Input: part model. Units: mm. Frame: model coordinates. A direction names the side the tool comes from. Round coordinates to 2 decimals unless told otherwise and drop trailing zeros. Loops run counter-clockwise (first coordinate to the right, second up) from the corner with the lowest first, then second, coordinate; pieces in that order, holes last.
1) Section A-A, the plane y = 34. Return loops of the section in (x, z).
2) Section C-C, the plane z = 18. Return loops of the section in (x, y), and give its area (3 significant figures).
3) Access query for faces 1 (the face through (6, 24, 7.5)), 2 (the face through (2, 22.7, -14.4)). Directions: +Z, -Z, +X, -X, +Y, -Y. A direction counts if a zero-diameter tool reaches every point of the face in a straight line with its end or side. Return the directions, or none.
4) First-contact query: pin 1 (1.5 mm diameter, centred on y = 36, z = -18.5, fed in from +X); pin 2 (6 mm diameter, centred on y = 25, z = 19.5, fed in from -X); pin 3 (10 mm diameter, centred on y = 11, z = -16, fed in from +X); pin 4 (10 mm diameter, centred on y = 15, z = -1, fed in from -X). Flat tips, straight axial feed; report the tip coordinate or a pass-through.
5) Section B-B, the plane x = 0. Return loops of the section in (y, z), and give its area (3 significant figures).
6) Ray query, line 1 along Y through (x, z) = (0, -16); line 2 along Z through (x, y) = (-9.5, 23); line 3 along Z through (x, y) = (-19, 27.5). Return the intervals inside material, ascending.
7) Draft query along Z for faces 3 (the face through (7.509, 9.86, 23.846)), 4 (the face through (0, 0, 0)), 5 (the face through (6, 24, -7.5)), 6 (the face through (0, 20, 0)). Return one class per face: pulls with the +Z half, pulls with the -Z half, needs draft (parallel to the pull), parting line crosses it, or undercut.
8) Section D-D, the plane y = 27. Return loops of the section in (x, z), and give its area (3 significant figures).
from build123d import *

# Parameters (mm, degrees)
SKETCH1_R               = 25
BOSS_EXTRUDE1_DEPTH     = 20
SKETCH5_W               = 7.5
SKETCH5_H               = 25.626943466
CUT_EXTRUDE1_DEPTH      = 25
CUT_EXTRUDE2_DEPTH      = 25
CUT_EXTRUDE2_DEPTH_BACK = 25
SKETCH6_R               = 10


with BuildPart() as part:
    # Sketch1 → Boss-Extrude1 (new body)
    with BuildSketch(Plane(origin=(0, 0, 0), x_dir=(1, 0, 0), z_dir=(0, 1, 0))):
        with Locations(Location((0, 0, 0), (0, 0, 270))):
            Circle(SKETCH1_R)
    extrude(amount=BOSS_EXTRUDE1_DEPTH)

    # Sketch4 → Revolve1 (revolve)
    with BuildSketch(Plane.XY):
        with BuildLine():
            Line((0, 45), (0, 20))
            Line((0, 20), (25, 20))
            ThreePointArc((25, 20), (17.67766953, 37.67766953), (0, 45))
        make_face()
    revolve(axis=Axis((0, 45, 0), (0, -1, 0)))

    # Sketch5 → Cut-Extrude1 (cut, symmetric)
    with BuildSketch(Plane(origin=(0, 0, 0), x_dir=(0, 0, -1), z_dir=(1, 0, 0))):
        with Locations((3.75, 32.813471733)):
            Rectangle(SKETCH5_W, SKETCH5_H)
    cut_extrude1 = extrude(amount=CUT_EXTRUDE1_DEPTH, both=True, mode=Mode.SUBTRACT)

    # Mirror1: Cut-Extrude1 across plane
    add(cut_extrude1.mirror(Plane.XY), mode=Mode.SUBTRACT)

    # Sketch6 → Cut-Extrude2 (cut, two sides: drawn at the far end of the back side and taken through both)
    with BuildSketch(Plane.XY.offset(-CUT_EXTRUDE2_DEPTH_BACK)):
        with Locations(Location((0, 32.5, 0), (0, 0, 223.948453445))):
            Circle(SKETCH6_R)
    extrude(amount=CUT_EXTRUDE2_DEPTH + CUT_EXTRUDE2_DEPTH_BACK, mode=Mode.SUBTRACT)


solid = part.part
Final values:
1. outline: (-19.31, -7.5) arc R20.71 ccw to (-9.89, -18.2) - (-9.89, -7.5) - close; (-19.31, 7.5) - (-9.89, 7.5) - (-9.89, 18.2) arc R20.71 ccw to start; (9.89, -18.2) arc R20.71 ccw to (19.31, -7.5) - (9.89, -7.5) - close; (9.89, 7.5) - (19.31, 7.5) arc R20.71 ccw to (9.89, 18.2) - close
2. outline: (-17.35, 0) - (17.35, 0) - (17.35, 20) arc R17.35 ccw to (9.84, 34.29) arc R10 cw (long way) to (-9.84, 34.29) arc R17.35 ccw to (-17.35, 20) - close
2. area: 933 mm2
3. face 1: +X, -X, +Y
3. face 2: +Z, -Z
4. pin 1: passes through
4. pin 2: stops at x = -18.21
4. pin 3: stops at x = 22.45
4. pin 4: stops at x = -25
5. outline: (0, -25) - (20, -25) arc R25 ccw to (22.5, -24.87) - (22.5, -7.5) - (20, -7.5) - (20, 7.5) - (22.5, 7.5) - (22.5, 24.87) arc R25 ccw to (20, 25) - (0, 25) - close; (42.5, -10.9) arc R25 ccw to (43.85, -7.5) - (42.5, -7.5) - close; (42.5, 7.5) - (43.85, 7.5) arc R25 ccw to (42.5, 10.9) - close
5. area: 1,090 mm2
6. line 1: y = 0 to 22.5
6. line 2: z = -22.93 to -7.5, 7.5 to 22.93
6. line 3: z = -14.41 to -7.5, 7.5 to 14.41
7. face 3: parting line crosses it
7. face 4: needs draft
7. face 5: undercut
7. face 6: undercut
8. outline: (-22.8, -7.5) arc R24 ccw to (-8.35, -22.5) - (-8.35, -7.5) - close; (-22.8, 7.5) - (-8.35, 7.5) - (-8.35, 22.5) arc R24 ccw to start; (8.35, -22.5) arc R24 ccw to (22.8, -7.5) - (8.35, -7.5) - close; (8.35, 7.5) - (22.8, 7.5) arc R24 ccw to (8.35, 22.5) - close
8. area: 567 mm2
